from build123d import *

# Parameters (mm, degrees)
SALIENTE_EXTRUIR1_DEPTH = 2.5


with BuildPart() as part:
    # Croquis1 → Saliente-Extruir1 (new body)
    with BuildSketch(Plane.XY):
        with BuildLine():
            Line((-16.5, -88), (-12.5, -88))
            Line((-12.5, -88), (-12.5, -57.1))
            Line((-12.5, -57.1), (12.5, -57.1))
            Line((12.5, -57.1), (12.5, -88))
            Line((12.5, -88), (16.5, -88))
            Line((16.5, -88), (28.350564417, -20.2223184))
            ThreePointArc((28.350564417, -20.2223184), (28.462571058, -19.364394538), (28.5, -18.5))
            Line((28.5, -18.5), (28.5, 18.5))
            ThreePointArc((28.5, 18.5), (25.571067812, 25.571067812), (18.5, 28.5))
            Line((18.5, 28.5), (-18.5, 28.5))
            ThreePointArc((-18.5, 28.5), (-25.571067812, 25.571067812), (-28.5, 18.5))
            Line((-28.5, 18.5), (-28.5, -18.5))
            ThreePointArc((-28.5, -18.5), (-28.462571058, -19.364394538), (-28.350564417, -20.2223184))
            Line((-28.350564417, -20.2223184), (-16.5, -88))
        make_face()
    extrude(amount=SALIENTE_EXTRUIR1_DEPTH)


solid = part.part
Part model, mm, in its own coordinate system. A direction names the side the tool comes from. Coordinates: 2 decimals unless noted, no trailing zeros. Loops run counter-clockwise (first coordinate to the right, second up) from the corner with the lowest first, then second, coordinate; pieces in that order, holes last. Notation, with made-up numbers: M -1.5,12.5 L 31.5,12.5 A14 ccw 31.5,28.5 Z; hole C 82,-4 d6. An arc over 180 degrees is marked long. Use a Markdown table: item, result. Add a question column.
Q1. Cut at B-B (y = -63). Write the cut outline in (x, z).
Q2. Pin check, flat tips, straight feed: P1, Ø1.5, axis at y = -28, z = 1, coming from the +X side; P2, Ø1.5, axis at y = -70.5, z = 2, coming from the +X side; P3, Ø0.8, axis at x = 1.5, z = 1.5, coming from the -Y side. Stop position of each tip, or through.
Q3. Probe L1, parallel to Y at x = 11, z = 0.4; L2, parallel to X at y = -58, z = 1.35; L3, parallel to X at y = -69, z = 2.15. List the from-to ranges inside material, lowest first.
Q4. Cut at D-D (y = -34.5). Write the cut outline in (x, z), and give its area (3 significant figures).
Q5. Cut at C-C (x = -7). Write the cut outline in (y, z).
Q6. Which spindle directions (+Z, -Z, +X, -X, +Y, -Y) get a long thin tool onto all of the face, cutting with end or side? Do faces 1 (the cylindrical face through (-25.49, 25.65, 1.23)), 2 (the flat face through (-12.5, -73, 1)). Say none if no direction does.
Q7. Cut at A-A (z = 1.8). Write the cut outline in (x, y).
Worked out:
| question | item | result |
|---|---|---|
| 1 | outline | M -20.87,0 L -12.5,0 L -12.5,2.5 L -20.87,2.5 Z; M 12.5,0 L 20.87,0 L 20.87,2.5 L 12.5,2.5 Z |
| 2 | P1 | stops at x = 27.12 |
| 2 | P2 | stops at x = 19.69 |
| 2 | P3 | stops at y = -57.1 |
| 3 | L1 | y = -57.1 to 28.5 |
| 3 | L2 | x = -21.75 to -12.5, 12.5 to 21.75 |
| 3 | L3 | x = -19.82 to -12.5, 12.5 to 19.82 |
| 4 | outline | M -25.85,0 L 25.85,0 L 25.85,2.5 L -25.85,2.5 Z |
| 4 | area | 129 mm2 |
| 5 | outline | M -57.1,0 L 28.5,0 L 28.5,2.5 L -57.1,2.5 Z |
| 6 | face 1 | +Z, -Z, -X, +Y |
| 6 | face 2 | +Z, -Z, -Y |
| 7 | outline | M -28.5,-18.5 A10 ccw -28.35,-20.22 L -16.5,-88 L -12.5,-88 L -12.5,-57.1 L 12.5,-57.1 L 12.5,-88 L 16.5,-88 L 28.35,-20.22 A10 ccw 28.5,-18.5 L 28.5,18.5 A10 ccw 18.5,28.5 L -18.5,28.5 A10 ccw -28.5,18.5 Z |
